```python
from build123d import *

# Parameters (mm, degrees)
F0_W     = 50
F0_H     = 50
F1_DEPTH = 4
F2_W     = 43.4
F2_H     = 43.4
F3_DEPTH = 3
F4_R     = 3
F4_R_2   = 10
F5_DEPTH = 25
F7_DEPTH = 3
F8_R     = 3


with BuildPart() as f1:
    # F0 (on Front) → F1 (new body)
    with BuildSketch(Plane.XZ):
        Rectangle(F0_W, F0_H)
    extrude(amount=-F1_DEPTH)

    # F2 (on face) → F3 (join)
    with BuildSketch(Plane(origin=(0, 4, 0), x_dir=(-1, 0, 0), z_dir=(0, 1, 0))):
        Rectangle(F2_W, F2_H)
    extrude(amount=F3_DEPTH)

    # F4 (on face) → F5 (cut)
    with BuildSketch(Plane(origin=(0, 7, 0), x_dir=(-1, 0, 0), z_dir=(0, 1, 0))):
        with Locations((-16.5, 16.5)):
            Circle(F4_R)
        with Locations((16.5, 16.5)):
            Circle(F4_R)
        with Locations((16.5, -16.5)):
            Circle(F4_R)
        with Locations((-16.5, -16.5)):
            Circle(F4_R)
        Circle(F4_R_2)
    extrude(amount=-F5_DEPTH, mode=Mode.SUBTRACT)

    # F6 (on face) → F7 (cut)
    with BuildSketch(Plane.XZ):
        Polygon((-19.386751, 11.5), (-13.613249, 11.5), (-10.726497, 16.5), (-13.613249, 21.5), (-19.386751, 21.5), (-22.273503, 16.5), align=None)
        Polygon((19.386751, 21.5), (13.613249, 21.5), (10.726497, 16.5), (13.613249, 11.5), (19.386751, 11.5), (22.273503, 16.5), align=None)
        Polygon((13.613249, -21.5), (19.386751, -21.5), (22.273503, -16.5), (19.386751, -11.5), (13.613249, -11.5), (10.726497, -16.5), align=None)
        Polygon((-19.386751, -21.5), (-13.613249, -21.5), (-10.726497, -16.5), (-13.613249, -11.5), (-19.386751, -11.5), (-22.273503, -16.5), align=None)
    extrude(amount=-F7_DEPTH, mode=Mode.SUBTRACT)

    # F8
    f8_edges = [f1.edges().sort_by_distance(p)[0] for p in [
        (21.7, 5.5, 21.7),
        (-21.7, 5.5, 21.7),
        (-21.7, 5.5, -21.7),
        (21.7, 5.5, -21.7),
    ]]
    fillet(f8_edges, radius=F8_R)


solid = f1.part
```
Verification items for the finished model (mm, model axes). A direction names the side the tool comes from. Coordinates: 2 decimals unless noted, no trailing zeros. Loops run counter-clockwise (first coordinate to the right, second up) from the corner with the lowest first, then second, coordinate; pieces in that order, holes last. Notation, with made-up numbers: (44, -9.75) -> (102, -9.75) arc R18 ccw to (102, 10.25) -> close; hole circle Ø6 at (53.25, 58.25). An arc over 180 degrees is marked (long way). Answer in a Markdown table with one row per item.
1) Depth check by flat-ended pin: P1, Ø1.5, axis at y = 6, z = -16.5, coming from the -X side; P2, Ø5, axis at x = 15.5, z = 15.5, coming from the -Y side; P3, Ø1, axis at x = -7, y = 5, coming from the -Z side. Enter the tip coordinate at first touch or a pass-through.
The answers:
| item | result |
|---|---|
| P1 | stops at x = -21.7 |
| P2 | stops at y = 3 |
| P3 | stops at z = -21.7 |
2) Scan lines: line 1 along Z through (x, y) = (-16.5, 5.7); line 2 along Z through (x, y) = (-14, 6.5); line 3 along X through (y, z) = (0.75, 14). Record each from-to range of solid material in increasing order. Write a range as from..to.
The answers:
| item | result |
|---|---|
| line 1 | z = -21.7..-19.5, -13.5..13.5, 19.5..21.7 |
| line 2 | z = -21.7..-18.16, -14.84..14.84, 18.16..21.7 |
| line 3 | x = -25..-20.83, -12.17..12.17, 20.83..25 |
3) Access from +Z, -Z, +X, -X, +Y, -Y to the whole of each face (thin tool, end or side, straight path). Record for faces 1 (the face through (-20.84, 5.52, -20.8)), 2 (the face through (12.19, 1.479, -13.965)), 3 (the face through (-23, 4, 0)).
The answers:
| item | result |
|---|---|
| face 1 | -Z, -X, +Y |
| face 2 | -Y |
| face 3 | +Y |
4) Section check D-D (x = -16.5). Record the cut outline in (y, z), and give its area (3 significant figures).
The answers:
| item | result |
|---|---|
| outline | (0, -25) -> (4, -25) -> (4, -21.7) -> (7, -21.7) -> (7, -19.5) -> (3, -19.5) -> (3, -21.5) -> (0, -21.5) -> close; (0, -11.5) -> (3, -11.5) -> (3, -13.5) -> (7, -13.5) -> (7, 13.5) -> (3, 13.5) -> (3, 11.5) -> (0, 11.5) -> close; (0, 21.5) -> (3, 21.5) -> (3, 19.5) -> (7, 19.5) -> (7, 21.7) -> (4, 21.7) -> (4, 25) -> (0, 25) -> close |
| area | 222 mm2 |
5) Section check C-C (z = -5). Record the cut outline in (x, y).
The answers:
| item | result |
|---|---|
| outline | (-25, 0) -> (-8.66, 0) -> (-8.66, 7) -> (-21.7, 7) -> (-21.7, 4) -> (-25, 4) -> close; (8.66, 0) -> (25, 0) -> (25, 4) -> (21.7, 4) -> (21.7, 7) -> (8.66, 7) -> close |
6) Section check B-B (x = 6). Record the cut outline in (y, z).
The answers:
| item | result |
|---|---|
| outline | (0, -25) -> (4, -25) -> (4, -21.7) -> (7, -21.7) -> (7, -8) -> (0, -8) -> close; (0, 8) -> (7, 8) -> (7, 21.7) -> (4, 21.7) -> (4, 25) -> (0, 25) -> close |
7) Draft check along Z on faces 4 (the face through (-25, 2, 0)), 5 (the face through (20.84, 5.52, -20.8)), 6 (the face through (-14, 3, 19)). Enter one of: released by +Z, released by -Z, zero draft, split by the parting line, or undercut.
The answers:
| item | result |
|---|---|
| face 4 | zero draft |
| face 5 | released by -Z |
| face 6 | undercut |
8) Section check A-A (y = 5.5). Record the cut outline in (x, z), and give its area (3 significant figures).
The answers:
| item | result |
|---|---|
| outline | (-21.7, -18.7) arc R3 ccw to (-18.7, -21.7) -> (18.7, -21.7) arc R3 ccw to (21.7, -18.7) -> (21.7, 18.7) arc R3 ccw to (18.7, 21.7) -> (-18.7, 21.7) arc R3 ccw to (-21.7, 18.7) -> close; hole circle Ø6 at (-16.5, -16.5); hole circle Ø6 at (-16.5, 16.5); hole circle Ø20 at (0, 0); hole circle Ø6 at (16.5, -16.5); hole circle Ø6 at (16.5, 16.5) |
| area | 1,450 mm2 |
